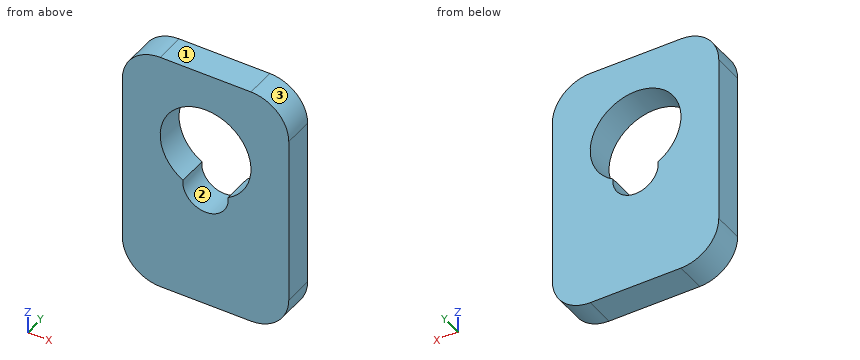
```python
from build123d import *

# Parameters (mm, degrees)
F1_W     = 22
F1_H     = 32.5
F2_DEPTH = 4
F3_DEPTH = 4.001
F4_R     = 5


with BuildPart() as f2:
    # F1 (on Front) → F2 (new body)
    with BuildSketch(Plane.XZ):
        with Locations((0, -5.25)):
            Rectangle(F1_W, F1_H)
    extrude(amount=F2_DEPTH)

    # F0 (on Front) → F3 (cut, through all)
    with BuildSketch(Plane.XZ):
        with BuildLine():
            ThreePointArc((-2.985416, -5.204545), (0, -8.5), (2.985416, -5.204545))
            ThreePointArc((2.985416, -5.204545), (0, 6), (-2.985416, -5.204545))
        make_face()
    extrude(amount=F3_DEPTH, mode=Mode.SUBTRACT)

    # F4
    f4_edges = [f2.edges().sort_by_distance(p)[0] for p in [
        (11, -2, 11),
        (-11, -2, 11),
        (-11, -2, -21.5),
        (11, -2, -21.5),
    ]]
    fillet(f4_edges, radius=F4_R)


solid = f2.part
```
For this review, take the finished solid that the model builds, in its own axes (mm). Face numbers are marked on the shaded views. Round coordinates to 2 decimals unless told otherwise and drop trailing zeros. Loops run counter-clockwise (first coordinate to the right, second up) from the corner with the lowest first, then second, coordinate; pieces in that order, holes last.
Q1. Mouldability with a two-part tool opening along X and no side actions: class the marked faces 1, 2 and 3 as +X half, -X half, draft (parallel to the pull), parting line (faces both ways), or undercut.
Result sheet:
face 1: draft
face 2: undercut
face 3: +X half
Q2. Add section C-C on y = -0.8. Write out the cut boundary in (x, z), plus the area to 3 significant figures.
Result sheet:
outline: (-11, -16.5) arc R5 ccw to (-6, -21.5) - (6, -21.5) arc R5 ccw to (11, -16.5) - (11, 6) arc R5 ccw to (6, 11) - (-6, 11) arc R5 ccw to (-11, 6) - close; hole (-2.99, -5.2) arc R3 ccw (long way) to (2.99, -5.2) arc R6 ccw (long way) to start
area: 568 mm2
Q3. To check wall thickness, follow line 1 along Z through (x, y) = (0, -1.1); line 2 along X through (y, z) = (-1.95, -5.5); line 3 along X through (y, z) = (-1.1, 0). State the ranges of each line that lie inside material, in increasing order.
Result sheet:
line 1: z = -21.5 to -8.5, 6 to 11
line 2: x = -11 to -3, 3 to 11
line 3: x = -11 to -6, 6 to 11
Q4. Insertion check: pin 1 Ø1 at (x, y) = (8.5, -3.5) entering from +Z. The pin has a flat end and moves straight along its axis. Give the tip position at first contact, or say it passes through.
Result sheet:
pin 1: stops at z = 10.58
Q5. Add section A-A on z = 0. Write out the cut boundary in (x, y).
Result sheet:
outline: (-11, -4) - (-6, -4) - (-6, 0) - (-11, 0) - close; (6, -4) - (11, -4) - (11, 0) - (6, 0) - close
Q6. Add section B-B on x = 0. Write out the cut boundary in (y, z).
Result sheet:
outline: (-4, -21.5) - (0, -21.5) - (0, -8.5) - (-4, -8.5) - close; (-4, 6) - (0, 6) - (0, 11) - (-4, 11) - close
